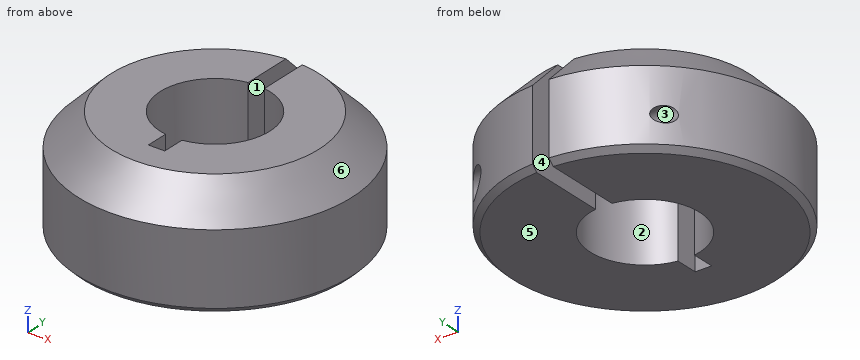
from build123d import *

# Parameters (mm, degrees)
BOSS_EXTRUDE1_DEPTH = 10
CHAMFER1_SIZE       = 3
CHAMFER2_SIZE       = 0.5
SKETCH22_R          = 1.225
CUT_EXTRUDE1_DEPTH  = 10
SKETCH23_R          = 0.725
CUT_EXTRUDE2_DEPTH  = 27.7500001


with BuildPart() as part:
    # Sketch1 → Boss-Extrude1 (new body)
    with BuildSketch(Plane.XY):
        with BuildLine():
            Line((-0.75, 4.943429983), (-0.75, 12.477479713))
            ThreePointArc((-0.75, 12.477479713), (0, -12.5), (0.75, 12.477479713))
            Line((0.75, 12.477479713), (0.75, 4.943429983))
            ThreePointArc((0.75, 4.943429983), (5, 0), (0.75, -4.943429983))
            Line((0.75, -4.943429983), (0.75, -7))
            Line((0.75, -7), (-0.75, -7))
            Line((-0.75, -7), (-0.75, -4.943429983))
            ThreePointArc((-0.75, -4.943429983), (-5, 0), (-0.75, 4.943429983))
        make_face()
    extrude(amount=BOSS_EXTRUDE1_DEPTH)

    # Chamfer1
    chamfer1_edges = [part.edges().sort_by_distance(p)[0] for p in [
        (0, -12.5, 10),
    ]]
    chamfer(chamfer1_edges, length=CHAMFER1_SIZE)

    # Chamfer2
    chamfer2_edges = [part.edges().sort_by_distance(p)[0] for p in [
        (0, -12.5, 0),
    ]]
    chamfer(chamfer2_edges, length=CHAMFER2_SIZE)

    # Sketch22 → Cut-Extrude1 (cut)
    with BuildSketch(Plane(origin=(14.25, 0, 0), x_dir=(0, 0, -1), z_dir=(1, 0, 0))):
        with Locations((-3, 9)):
            Circle(SKETCH22_R)
    extrude(amount=-CUT_EXTRUDE1_DEPTH, mode=Mode.SUBTRACT)

    # Sketch23 → Cut-Extrude2 (cut, through all)
    with BuildSketch(Plane(origin=(14.25, 0, 0), x_dir=(0, 0, -1), z_dir=(1, 0, 0))):
        with Locations((-3, 9)):
            Circle(SKETCH23_R)
    extrude(amount=-CUT_EXTRUDE2_DEPTH, mode=Mode.SUBTRACT)


solid = part.part
Here's how the part is built. I have some questions about the finished solid (model axes, mm). Face numbers are marked on the shaded views. A direction names the side the tool comes from. Coordinates: 2 decimals unless noted, no trailing zeros. Write each loop counter-clockwise with the first axis right and the second up, starting at its lowest first coordinate (ties: lowest second). Pieces come first, ordered by that corner, then holes.
Item 1: Will these pins go through, and if not, where does the flat tip stop? pin 1 (0.9 mm diameter, centred on y = 9, z = 3, fed in from -X); pin 2 (6 mm diameter, centred on y = 8.5, z = 2, fed in from -X) (3 decimals); pin 3 (1 mm diameter, centred on x = 2.5, y = 4.5, fed in from -Z); pin 4 (1.5 mm diameter, centred on y = 2.5, z = 2, fed in from -X).
Item 2: I want a section at C-C on x = 0. Write out the boundary of the cut face in (y, z).
Item 3: If we mould it in two halves opening along X, with no side actions, what happens to the marked faces 4, 5 and 6? For each: +X half, -X half, draft (parallel to the pull), parting line (faces both ways), or undercut.
Item 4: If I drill on line 1 (Y direction, x = 2, z = 3.25); line 2 (Y direction, x = 3.2, z = 3) (3 decimals); line 3 (X direction, y = 7, z = 7.25), over which ranges is the centre line in solid material (lowest first)?
Item 5: I want a section at D-D on x = 3.5. Count the separate pieces of the cut face and the enclosed holes in it, and give its area (3 significant figures).
Item 6: I want a section at A-A on y = 0. Write out the boundary of the cut face in (x, z), and give its area (3 significant figures).
Item 7: I want a section at B-B on z = 4.75. Write out the boundary of the cut face in (x, y), and give its area (3 significant figures).
Item 8: On a 3-axis mill with a long thin cutter (end or side, diameter ignored), from which of +Z, -Z, +X, -X, +Y, -Y can I reach the whole of each face in a straight line? I mean the marked faces 1, 2 and 3. Say none if no direction works.
Findings below:
1. pin 1: passes through
1. pin 2: stops at x = -11.225
1. pin 3: stops at z = 0
1. pin 4: stops at x = -12.38
2. outline: (-12.5, 0.5) - (-12, 0) - (-7, 0) - (-7, 10) - (-9.5, 10) - (-12.5, 7) - close
3. face 4: undercut
3. face 5: draft
3. face 6: parting line
4. line 1: y = -12.34 to -4.58, 4.58 to 8.32, 9.68 to 12.34
4. line 2: y = -12.083 to -3.842, 3.842 to 8.275, 9.725 to 12.083
4. line 3: x = -10.05 to -0.75, 0.75 to 10.05
5. separate pieces: 2
5. enclosed holes: 1
5. area: 157 mm2
6. outline: (-12.5, 0.5) - (-12, 0) - (-5, 0) - (-5, 10) - (-9.5, 10) - (-12.5, 7) - close; (5, 0) - (12, 0) - (12.5, 0.5) - (12.5, 7) - (9.5, 10) - (5, 10) - close
6. area: 141 mm2
7. outline: (-0.75, -7) - (-0.75, -4.94) arc R5 cw to (-0.75, 4.94) - (-0.75, 12.48) arc R12.5 ccw (long way) to (0.75, 12.48) - (0.75, 4.94) arc R5 cw to (0.75, -4.94) - (0.75, -7) - close
7. area: 398 mm2
8. face 1: +Z, -Z, +Y
8. face 2: +Z, -Z
8. face 3: +X, -X
